Build history of the part. All positions in model axes, mm. Give positions to 0.01 mm unless a question says otherwise; leave off trailing zeros. Loops run counter-clockwise (first coordinate to the right, second up) from the corner with the lowest first, then second, coordinate; pieces in that order, holes last. Notation, with made-up numbers: M -12.5,30.5 L 3.5,30.5 A21 ccw 3.5,51.5 Z; hole C 3.25,20 d7. An arc over 180 degrees is marked long. Put each result on its own line as item: value.
```python
from build123d import *

# Parameters (mm, degrees)
FILLET1_R = 6.35


with BuildPart() as part:
    # Sketch2 → Revolve1 (revolve)
    with BuildSketch(Plane(origin=(0, 0, 0), x_dir=(0, 0, -1), z_dir=(1, 0, 0))):
        with BuildLine():
            Line((35.6108, 0), (44.3992, 0))
            ThreePointArc((44.3992, 0), (37.458984081, -34.604022474), (17.711827813, -63.8556))
            Line((17.711827813, -63.8556), (-44.3992, -63.8556))
            Line((-44.3992, -63.8556), (-44.3992, -57.3786))
            Line((-44.3992, -57.3786), (6.9088, -57.0357))
            Line((6.9088, -57.0357), (6.910792633, -57.0357))
            ThreePointArc((6.910792633, -57.0357), (11.868455582, -55.955071974), (15.926669287, -52.909241979))
            ThreePointArc((15.926669287, -52.909241979), (30.530340961, -28.226108874), (35.6108, 0))
        make_face()
    revolve(axis=Axis((0, 0, 44.3992), (0, 0, -1)))

    # Fillet1
    fillet1_edges = [part.edges().sort_by_distance(p)[0] for p in [
        (0, 63.8556, -17.711827813),
    ]]
    fillet(fillet1_edges, radius=FILLET1_R)


solid = part.part
```
Q1. Drop flat-ended pins along their axis: pin 1 Ø1 at (x, z) = (-14.5, 15.5) entering from +Y; pin 2 Ø2 at (y, z) = (29, -20) entering from -X; pin 3 Ø8 at (y, z) = (-13.5, -17) entering from -X. Give the stop position or say it passes through.
Here are the results:
pin 1: y = 62.3
pin 2: x = -55.47
pin 3: x = -63.08
Q2. Probe line 1 (X direction, y = 0, z = -6.85); line 2 (X direction, y = 44, z = 14.5). List the from-to ranges inside material, lowest first. Write a range as from..to.
Here are the results:
line 1: -63.86..-57.04, 57.04..63.86
line 2: -46.28..-36.52, 36.52..46.28
Q3. Mould opens along Y. For faces 1 (the flat face through (-23.95, 52.33, 44.399)), 2 (the conical face through (-17.183, -54.563, 18.386)), 3 (the cylindrical face through (-43.16, 47.06, 15.09)) say: pulls with the +Y half, pulls with the -Y half, needs draft (parallel to the pull), parting line crosses it, or undercut.
Here are the results:
face 1: needs draft
face 2: undercut
face 3: parting line crosses it
Q4. Slice it at A-A (z = 10). List the corners of the cut face in (x, y), and give its area (3 significant figures).
Here are the results:
outline: C 0,0 d127.71; hole C 0,0 d114.3
area: 2,550 mm²
Q5. Slice it at B-B (z = -23.5). List the corners of the cut face in (x, y), and give its area (3 significant figures).
Here are the results:
outline: C 0,0 d115.14; hole C 0,0 d85.18
area: 4,710 mm²
